Part model, mm, in its own coordinate system. A direction names the side the tool comes from. Give positions to 0.01 mm unless a question says otherwise; leave off trailing zeros. Loops run counter-clockwise (first coordinate to the right, second up) from the corner with the lowest first, then second, coordinate; pieces in that order, holes last. Notation, with made-up numbers: M 60.5,59 L 69.5,59 A15 ccw 69.5,70 Z; hole C 22,36 d5. An arc over 180 degrees is marked long. Put each result on its own line as item: value. Start each with the question number.
```python
from build123d import *

# Parameters (mm, degrees)
CORTAR_EXTRUIR1_START                       = 1
CROQUIS2_R                                  = 7.058141728
CORTAR_EXTRUIR1_DEPTH                       = 7
CHAFL_N1_SIZE                               = 0.1
DI_METRO_DE_TALADRO_1_0_1_1_D               = 1
DI_METRO_DE_TALADRO_1_0_1_1_DEPTH           = 0.2
DI_METRO_DE_TALADRO_1_0_1_1_TIP             = 0.30043031
DI_METRO_DE_TALADRO_1_0_1_1_ON_FACE_2_D     = 1
DI_METRO_DE_TALADRO_1_0_1_1_ON_FACE_2_DEPTH = 0.2
DI_METRO_DE_TALADRO_1_0_1_1_ON_FACE_2_TIP   = 0.30043031


with BuildPart() as part:
    # Croquis1 → Revolución1 (revolve)
    with BuildSketch(Plane.XY):
        with BuildLine():
            Line((0.2, 0), (0.25, 0))
            ThreePointArc((0.25, 0), (0.388524584, 0.03389675), (0.495745613, 0.127927069))
            Line((0.495745613, 0.127927069), (3.557104037, 4.5))
            Line((3.557104037, 4.5), (5.706019053, 4.5))
            Line((5.706019053, 4.5), (5.706019053, 7.568968696))
            Line((5.706019053, 7.568968696), (7.058141728, 9.5))
            Line((7.058141728, 9.5), (3, 9.5))
            Line((3, 9.5), (3, 15))
            Line((3, 15), (1.6, 15))
            Line((1.6, 15), (1.6, 2.799407209))
            Line((1.6, 2.799407209), (0.2, 0.8))
            Line((0.2, 0.8), (0.2, 0))
        make_face()
    revolve(axis=Axis((0, 0, 0), (0, 1, 0)))

    # Croquis2 → Cortar-Extruir1 (cut)
    with BuildSketch(Plane(origin=(0, 9.5, 0), x_dir=(1, 0, 0), z_dir=(0, 1, 0)).offset(CORTAR_EXTRUIR1_START)):
        Circle(CROQUIS2_R)
        Polygon((2.309401077, 4), (-2.309401077, 4), (-4.618802154, 0), (-2.309401077, -4), (2.309401077, -4), (4.618802154, 0), align=None, mode=Mode.SUBTRACT)
    extrude(amount=-CORTAR_EXTRUIR1_DEPTH, mode=Mode.SUBTRACT)

    # Chaflán1
    chafl_n1_edges = [part.edges().sort_by_distance(p)[0] for p in [
        (-1.6, 15, 0),
    ]]
    chamfer(chafl_n1_edges, length=CHAFL_N1_SIZE)

    # Diámetro de taladro Ø1.0 (1)1
    with Locations(Plane(origin=(3.464101615, 7, 2), x_dir=(-0.5, 0, 0.866025404), z_dir=(0.866025404, 0, 0.5))):
        with Locations((0, 0)):
            Hole(DI_METRO_DE_TALADRO_1_0_1_1_D / 2, depth=DI_METRO_DE_TALADRO_1_0_1_1_DEPTH)
            with Locations((0, 0, -(DI_METRO_DE_TALADRO_1_0_1_1_DEPTH + DI_METRO_DE_TALADRO_1_0_1_1_TIP / 2))):  # 118° drill point
                Cone(0, DI_METRO_DE_TALADRO_1_0_1_1_D / 2, DI_METRO_DE_TALADRO_1_0_1_1_TIP, mode=Mode.SUBTRACT)

    # Diámetro de taladro Ø1.0 (1)1 on face 2
    with Locations(Plane(origin=(0, 7, 4), x_dir=(1, 0, 0), z_dir=(0, 0, 1))):
        with Locations((0, 0)):
            Hole(DI_METRO_DE_TALADRO_1_0_1_1_ON_FACE_2_D / 2, depth=DI_METRO_DE_TALADRO_1_0_1_1_ON_FACE_2_DEPTH)
            with Locations((0, 0, -(DI_METRO_DE_TALADRO_1_0_1_1_ON_FACE_2_DEPTH + DI_METRO_DE_TALADRO_1_0_1_1_ON_FACE_2_TIP / 2))):  # 118° drill point
                Cone(0, DI_METRO_DE_TALADRO_1_0_1_1_ON_FACE_2_D / 2, DI_METRO_DE_TALADRO_1_0_1_1_ON_FACE_2_TIP, mode=Mode.SUBTRACT)


solid = part.part
```
1) Band-saw the part on B-B on y = 13. Give the cut face in (x, z).
2) Wall check: L1, parallel to X at y = 11.5, z = 0; L2, parallel to Y at x = 0, z = 3.95. Give the ranges that are in metal, low to high.
3) Which spindle directions (+Z, -Z, +X, -X, +Y, -Y) get a long thin tool onto all of the face, cutting with end or side? Do faces 4 (the flat face through (3.191, 7.591, 2.472)), 5 (the flat face through (3, 9.5, -1)), 6 (the flat face through (-3.4, 4.5, -1.5)), 7 (the flat face through (0, 15, 2)), 8 (the conical face through (3.056, 7.077, 1.811)). Say none if no direction does.
4) Pin check, flat tips, straight feed: pin 1 Ø2 at (y, z) = (13.5, -1.5) entering from +X; pin 2 Ø1.5 at (y, z) = (7.5, -1) entering from -X; pin 3 Ø1.5 at (x, z) = (-1, 3) entering from -Y (3 decimals). Stop position of each tip, or through.
5) Band-saw the part on A-A on y = 5.25. Give the cut face in (x, z), then the cut area to 3 significant figures.
6) Mould opens along Z. For faces 1 (the conical face through (-0.296, 1.373, 1.335)), 2 (the conical face through (-0.46, 1.34, 0.35)), 3 (the flat face through (3.48, 7.04, -1.97)) say: +Z half, -Z half, draft (parallel to the pull), parting line (faces both ways), or undercut.
7) Band-saw the part on C-C on y = 3.5. Give the cut face in (x, z).
Evaluation:
1. outline: C 0,0 d6; hole C 0,0 d3.2
2. L1: -3 to -1.6, 1.6 to 3
2. L2: 4.5 to 6.5, 7.5 to 9.5
3. face 4: +Z, +X, +Y, -Y
3. face 5: +Y
3. face 6: -Y
3. face 7: +Z, -Z, +X, -X, +Y
3. face 8: none
4. pin 1: x = 2.96
4. pin 2: x = -4.47
4. pin 3: y = 2.865
5. outline: M -4.62,0 L -2.31,-4 L 2.31,-4 L 4.62,0 L 2.31,4 L -2.31,4 Z; hole C 0,0 d3.2
5. area: 47.4 mm2
6. face 1: parting line
6. face 2: undercut
6. face 3: -Z half
7. outline: C 0,0 d5.71; hole C 0,0 d3.2
